Part print with two shaded views. Sizes in mm from the minimum x, y, z corner. Give positions to 0.01 mm unless a question says otherwise; leave off trailing zeros. Write each loop counter-clockwise with the first axis right and the second up, starting at its lowest first coordinate (ties: lowest second). Pieces come first, ordered by that corner, then holes. Notation, with made-up numbers: (-36.75, -40) - (16.25, -40) arc R24 ccw to (16.25, -26) - close; hole circle Ø4 at (44, 44). An arc over 180 degrees is marked (long way). Answer as a JSON object with one key per item and string values.
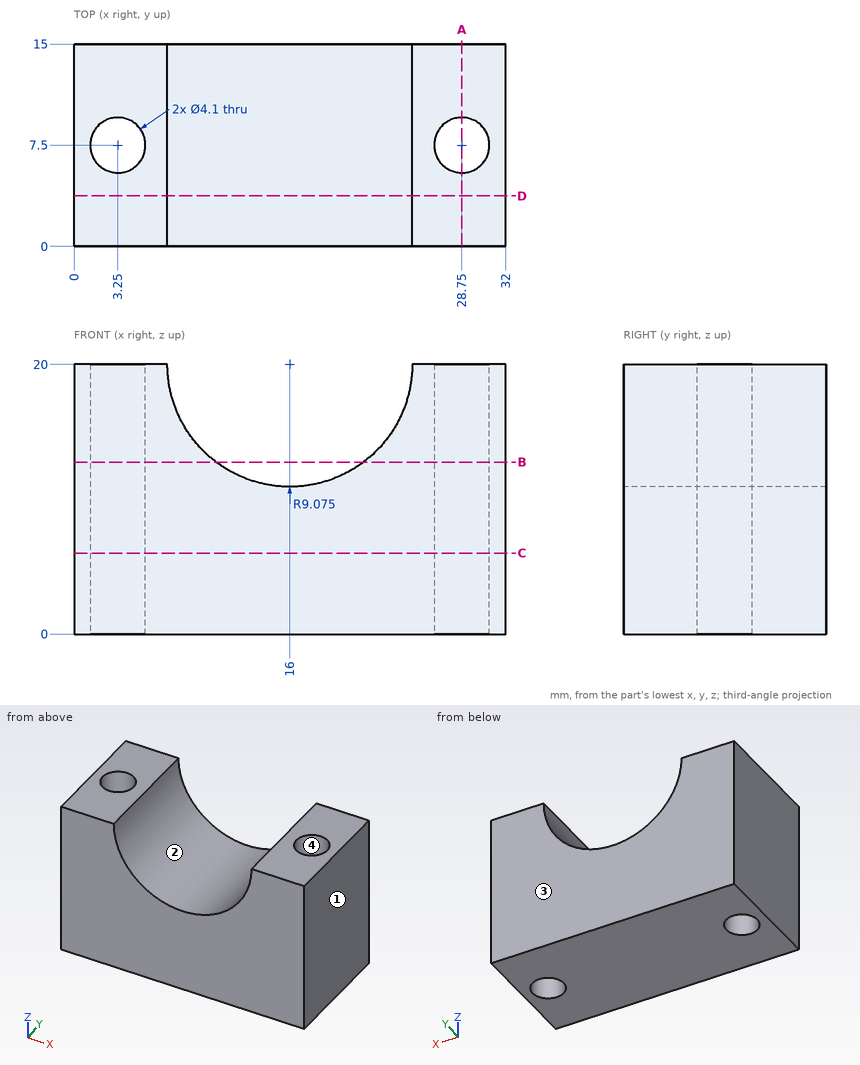
(1) Saw through at B-B, the plane z = 12.75. Give the cut face in (x, y), and give its area (3 significant figures).
Answer key:
{"outline": "(0, 0) - (10.54, 0) - (10.54, 15) - (0, 15) - close; (21.46, 0) - (32, 0) - (32, 15) - (21.46, 15) - close; hole circle Ø4.1 at (3.25, 7.5); hole circle Ø4.1 at (28.75, 7.5)", "area": "290 mm²"}
(2) Probe L1, parallel to X at y = 7.5, z = 8.75; L2, parallel to Y at x = 3.25, z = 13; L3, parallel to X at y = 0.5, z = 19. List the from-to ranges inside material, lowest first. Write a range as [from, to].
Answer key:
{"L1": "x = [0, 1.2], [5.3, 26.7], [30.8, 32]", "L2": "y = [0, 5.45], [9.55, 15]", "L3": "x = [0, 6.98], [25.02, 32]"}
(3) Saw through at A-A, the plane x = 28.75. Give the cut face in (y, z), and give its area (3 significant figures).
Answer key:
{"outline": "(0, 0) - (5.45, 0) - (5.45, 20) - (0, 20) - close; (9.55, 0) - (15, 0) - (15, 20) - (9.55, 20) - close", "area": "218 mm²"}
(4) Pull direction X, two halves, no side cores. Call the marked faces 1, 2, 3 and 4: pulls with the +X half, pulls with the -X half, needs draft (parallel to the pull), parting line crosses it, or undercut.
Answer key:
{"face 1": "pulls with the +X half", "face 2": "undercut", "face 3": "needs draft", "face 4": "undercut"}
(5) Flat gauge pins, fed straight in: P1, Ø6, axis at x = 11, z = 7, coming from the -Y side; P2, Ø1.5, axis at x = 20.5, y = 5.5, coming from the +Z side. Where does each tip first touch, or does it go through?
Answer key:
{"P1": "stops at y = 0", "P2": "stops at z = 12.6"}
(6) Saw through at C-C, the plane z = 6. Give the cut face in (x, y).
Answer key:
{"outline": "(0, 0) - (32, 0) - (32, 15) - (0, 15) - close; hole circle Ø4.1 at (3.25, 7.5); hole circle Ø4.1 at (28.75, 7.5)"}
(7) Saw through at D-D, the plane y = 3.75. Give the cut face in (x, z) (3 decimals).
Answer key:
{"outline": "(0, 0) - (32, 0) - (32, 20) - (25.075, 20) arc R9.075 cw to (6.925, 20) - (0, 20) - close"}
